Build history of the part. All positions in model axes, mm. A direction names the side the tool comes from. Coordinates: 2 decimals unless noted, no trailing zeros. Loops run counter-clockwise (first coordinate to the right, second up) from the corner with the lowest first, then second, coordinate; pieces in that order, holes last. Notation, with made-up numbers: (-34, 50) - (-29, 50) arc R11 cw to (-29, 68) - close; hole circle Ø5 at (4.25, 6). An arc over 180 degrees is marked (long way). One line per item, written item: value.
```python
from build123d import *

# Parameters (mm, degrees)
F1_DEPTH = 330
F2_R     = 2.75
F3_DEPTH = 4.25
F4_R     = 1.675
F5_DEPTH = 2.201


with BuildPart() as f1:
    # F0 (on Front) → F1 (new body)
    with BuildSketch(Plane.XZ):
        Polygon((-4.45, 4), (-4.45, 0), (4.45, 0), (4.45, 4), (3.45, 4), (3.45, 4.95), (4.45, 4.95), (4.45, 6.45), (-4.45, 6.45), (-4.45, 4.95), (-3.45, 4.95), (-3.45, 4), align=None)
    extrude(amount=F1_DEPTH)

    # F2 (on face) → F3 (cut)
    with BuildSketch(Plane.XY.offset(6.45)):
        with Locations((0, -320)):
            Circle(F2_R)
        with Locations((0, -300)):
            Circle(F2_R)
        with Locations((0, -280)):
            Circle(F2_R)
    extrude(amount=-F3_DEPTH, mode=Mode.SUBTRACT)

    # F4 (on face) → F5 (cut, through all)
    with BuildSketch(Plane.XY.offset(2.2)):
        with Locations((0, -320)):
            Circle(F4_R)
    extrude(amount=-F5_DEPTH, mode=Mode.SUBTRACT)


solid = f1.part
```
Item 1: Cut at A-A, the plane y = -300. Write the cut outline in (x, z), then the cut area to 3 significant figures.
Check result:
outline: (-4.45, 0) - (4.45, 0) - (4.45, 4) - (3.45, 4) - (3.45, 4.95) - (4.45, 4.95) - (4.45, 6.45) - (2.75, 6.45) - (2.75, 2.2) - (-2.75, 2.2) - (-2.75, 6.45) - (-4.45, 6.45) - (-4.45, 4.95) - (-3.45, 4.95) - (-3.45, 4) - (-4.45, 4) - close
area: 32.1 mm^2
Item 2: Probe probe 1 along Y at (x, z) = (0, 3.7); probe 2 along X at (y, z) = (-320, 5.25); probe 3 along Z at (x, y) = (4, -16.5). List the from-to ranges inside material, lowest first. Write a range as from..to.
Check result:
probe 1: y = -330..-322.75, -317.25..-302.75, -297.25..-282.75, -277.25..0
probe 2: x = -4.45..-2.75, 2.75..4.45
probe 3: z = 0..4, 4.95..6.45
Item 3: Drop flat-ended pins along their axis: P1, Ø3, axis at x = -0.5, y = -278.5, coming from the +Z side; P2, Ø3.5, axis at x = 0, y = -320, coming from the +Z side. Give the stop position or say it passes through.
Check result:
P1: stops at z = 6.45
P2: stops at z = 2.2
Item 4: Pull direction X, two halves, no side cores. Call faces 1 (the face through (-0.596, -302.685, 4.355)), 2 (the face through (0, -300, 2.2)), 3 (the face through (0, -163, 6.45)): released by +X, released by -X, zero draft, split by the parting line, or undercut.
Check result:
face 1: undercut
face 2: undercut
face 3: zero draft
Item 5: Tool access for faces 4 (the face through (0, -163, 0)), 5 (the face through (0, -280, 2.2)): list every direction of +Z, -Z, +X, -X, +Y, -Y with a clear straight run to the whole face (end or side of a thin tool).
Check result:
face 4: -Z, +X, -X, +Y, -Y
face 5: +Z
